The figure shows three views and two pictorial views of one solid part (mm, origin at its lowest corner). Answer the questions. A direction names the side the tool comes from. Round coordinates to 2 decimals unless told otherwise and drop trailing zeros. Order: outer loops, then holes, each group sorted by start corner. A loop starts at its lowest first (then second) coordinate and runs counter-clockwise, first axis right, second up. Notation, with made-up numbers: (-23.5, 86) -> (-7.5, 86) arc R6 ccw to (-7.5, 97) -> close; hole circle Ø9 at (-28, 82). An arc over 180 degrees is marked (long way). One line per item, written item: value. Start each with the question number.
1. Section A-A (z = 15.85) is taken. Give the vertices of the cut face in (x, y), then the cut area to 3 significant figures.
2. Section C-C (y = 8.5) is taken. Give the vertices of the cut face in (x, z).
3. Section D-D (z = 10) is taken. Give the vertices of the cut face in (x, y).
4. Flat-ended cylindrical pins translate along their axes: pin 1 Ø12 at (y, z) = (33, 11) entering from +X; pin 2 Ø1 at (y, z) = (52, 28) entering from -X; pin 3 Ø2 at (x, y) = (20.5, 51) entering from +Z. Find the tip coordinate at first contact, or state that the pin passes through.
5. The mould has two halves that part along X. Classify the marked faces 1, 2 and 3: released by +X, released by -X, zero draft, split by the parting line, or undercut.
6. Section B-B (x = 15.85) is taken. Give the vertices of the cut face in (y, z).
7. Consider line 1 (X direction, y = 50, z = 15.85); line 2 (Z direction, x = 17.5, y = 38) (1 decimal). Determine where each line is inside the solid, lowest interval first.
8. For the marked faces 4 and 5, determine the directions among +Z, -Z, +X, -X, +Y, -Y from which every point of the face is accessible in a straight line to the end or side of a thin tool.
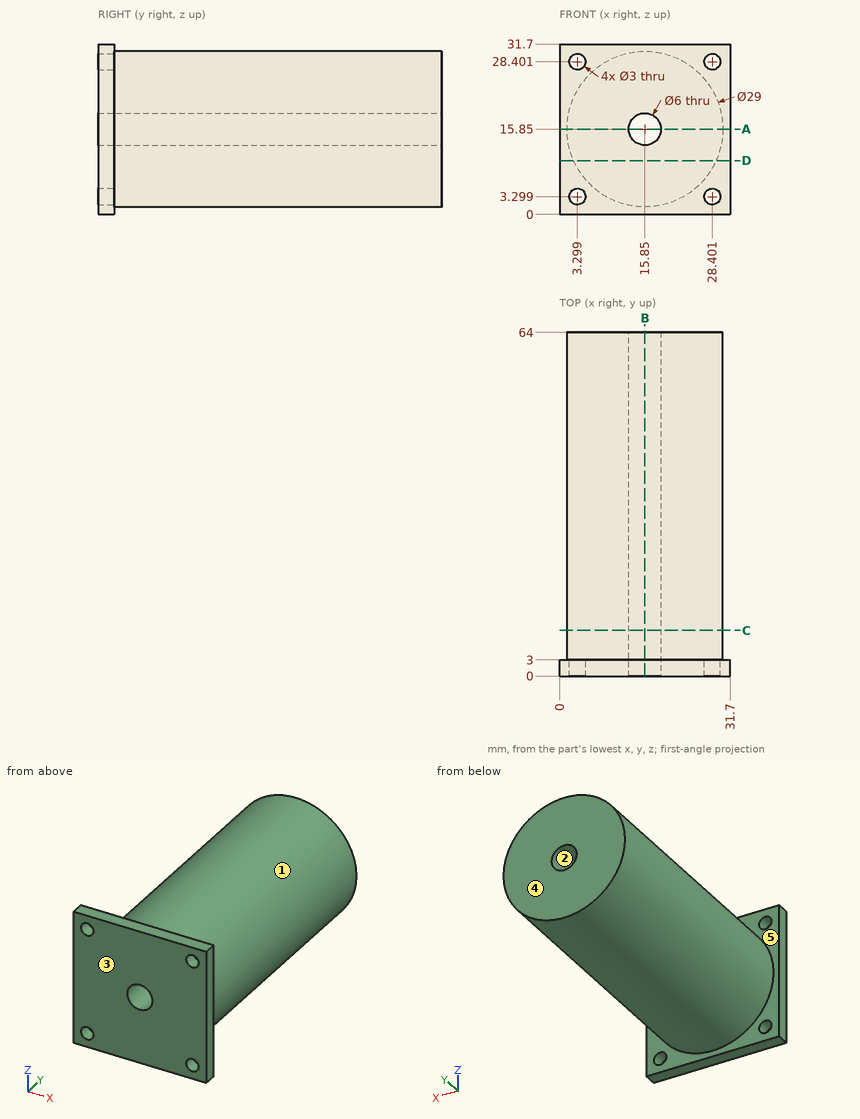
Answer:
1. outline: (0, 0) -> (12.85, 0) -> (12.85, 64) -> (1.35, 64) -> (1.35, 3) -> (0, 3) -> close; (18.85, 0) -> (31.7, 0) -> (31.7, 3) -> (30.35, 3) -> (30.35, 64) -> (18.85, 64) -> close
1. area: 1,480 mm^2
2. outline: circle Ø29 at (15.85, 15.85); hole circle Ø6 at (15.85, 15.85)
3. outline: (0, 0) -> (31.7, 0) -> (31.7, 3) -> (29.12, 3) -> (29.12, 64) -> (2.58, 64) -> (2.58, 3) -> (0, 3) -> close
4. pin 1: x = 30.35
4. pin 2: x = 7.22
4. pin 3: z = 29.88
5. face 1: split by the parting line
5. face 2: undercut
5. face 3: zero draft
6. outline: (0, 0) -> (3, 0) -> (3, 1.35) -> (64, 1.35) -> (64, 12.85) -> (0, 12.85) -> close; (0, 18.85) -> (64, 18.85) -> (64, 30.35) -> (3, 30.35) -> (3, 31.7) -> (0, 31.7) -> close
7. line 1: 1.35 to 12.85, 18.85 to 30.35
7. line 2: 1.4 to 13.3, 18.4 to 30.3
8. face 4: +Z, -Z, +X, -X, +Y
8. face 5: +Y
